```python
from build123d import *
from OCP.BRepFilletAPI import BRepFilletAPI_MakeChamfer

# Parameters (mm, degrees)
BOSS_EXTRUDE1_DEPTH = 37
CUT_EXTRUDE1_REACH  = 150.017
SKETCH2_W           = 42
SKETCH2_H           = 21
SKETCH3_R           = 2
CUT_EXTRUDE2_DEPTH  = 10
FILLET1_R           = 20
CUT_EXTRUDE5_REACH  = 150.017
SKETCH6_W           = 42
SKETCH6_H           = 9
SKETCH7_R           = 2
CUT_EXTRUDE6_DEPTH  = 10
CUT_EXTRUDE7_DEPTH  = 9
SKETCH9_R           = 2
CUT_EXTRUDE8_DEPTH  = 10
CUT_EXTRUDE9_DEPTH  = 6
SKETCH11_R          = 2
CUT_EXTRUDE10_DEPTH = 9
SKETCH12_R          = 2
CUT_EXTRUDE11_DEPTH = 10
CUT_EXTRUDE12_REACH = 140.091
CUT_EXTRUDE16_REACH = 142.222
SKETCH14_W          = 7
SKETCH14_H          = 27
CUT_EXTRUDE17_REACH = 108.34
SKETCH16_W          = 7
SKETCH16_H          = 10
CUT_EXTRUDE18_REACH = 146.306
SKETCH15_W          = 5
SKETCH15_H          = 10
CHAMFER1_SIZE       = 4.5
CHAMFER1_SIZE2      = 7.794228634
CUT_EXTRUDE19_DEPTH = 8


with BuildPart() as part:
    # Sketch1 → Boss-Extrude1 (new body)
    with BuildSketch(Plane(origin=(0, 0, 0), x_dir=(1, 0, 0), z_dir=(0, 1, 0))):
        Polygon((-15.317617866, 43.23325062), (45.682382134, 43.23325062), (45.682382134, -16.76674938), (65.682382134, -16.76674938), (65.682382134, 118.23325062), (45.682382134, 118.23325062), (45.682382134, 58.23325062), (-15.317617866, 58.23325062), align=None)
    extrude(amount=BOSS_EXTRUDE1_DEPTH)

    # Sketch2 → Cut-Extrude1 (cut, up to next)
    with BuildSketch(Plane(origin=(65.682382134, 0, 0), x_dir=(0, 0, -1), z_dir=(1, 0, 0)), mode=Mode.PRIVATE) as cut_extrude1_sk1:
        with Locations((13.23325062, 19.5)):
            Rectangle(SKETCH2_W, SKETCH2_H)
    cut_extrude1_tool1 = extrude(cut_extrude1_sk1.sketch, amount=-CUT_EXTRUDE1_REACH, mode=Mode.PRIVATE) & part.part
    # Sketch2 → Cut-Extrude1 (cut, up to next)
    with BuildSketch(Plane(origin=(65.682382134, 0, 0), x_dir=(0, 0, -1), z_dir=(1, 0, 0)), mode=Mode.PRIVATE) as cut_extrude1_sk2:
        with Locations((88.23325062, 19.5)):
            Rectangle(SKETCH2_W, SKETCH2_H)
    cut_extrude1_tool2 = extrude(cut_extrude1_sk2.sketch, amount=-CUT_EXTRUDE1_REACH, mode=Mode.PRIVATE) & part.part
    add(cut_extrude1_tool1.solids().sort_by_distance((65.682382, 19.5, -13.233251))[0], mode=Mode.SUBTRACT)
    add(cut_extrude1_tool2.solids().sort_by_distance((65.682382, 19.5, -88.233251))[0], mode=Mode.SUBTRACT)

    # Sketch3 → Cut-Extrude2 (cut)
    with BuildSketch(Plane.ZY.offset(-45.682382134)):
        with Locations((11.26674938, 24.75)):
            Circle(SKETCH3_R)
        with Locations((11.26674938, 15.25)):
            Circle(SKETCH3_R)
        with Locations((-37.73325062, 24.75)):
            Circle(SKETCH3_R)
        with Locations((-37.73325062, 15.25)):
            Circle(SKETCH3_R)
        with Locations(Location((-112.73325062, 24.75, 0), (0, 0, 180))):
            Circle(SKETCH3_R)
        with Locations(Location((-112.73325062, 15.25, 0), (0, 0, 180))):
            Circle(SKETCH3_R)
        with Locations(Location((-63.73325062, 15.25, 0), (0, 0, 180))):
            Circle(SKETCH3_R)
        with Locations(Location((-63.73325062, 24.75, 0), (0, 0, 180))):
            Circle(SKETCH3_R)
    extrude(amount=-CUT_EXTRUDE2_DEPTH, mode=Mode.SUBTRACT)

    # Fillet1
    fillet1_edges = [part.edges().sort_by_distance(p)[0] for p in [
        (55.682382134, 0, -118.23325062),
        (55.682382134, 0, 16.76674938),
    ]]
    fillet(fillet1_edges, radius=FILLET1_R)

    # Sketch6 → Cut-Extrude5 (cut, up to next)
    with BuildSketch(Plane(origin=(65.682382134, 0, 0), x_dir=(0, 0, -1), z_dir=(1, 0, 0)), mode=Mode.PRIVATE) as cut_extrude5_sk1:
        with Locations((13.23325062, 4.5)):
            Rectangle(SKETCH6_W, SKETCH6_H)
    cut_extrude5_tool1 = extrude(cut_extrude5_sk1.sketch, amount=-CUT_EXTRUDE5_REACH, mode=Mode.PRIVATE) & part.part
    # Sketch6 → Cut-Extrude5 (cut, up to next)
    with BuildSketch(Plane(origin=(65.682382134, 0, 0), x_dir=(0, 0, -1), z_dir=(1, 0, 0)), mode=Mode.PRIVATE) as cut_extrude5_sk2:
        with Locations((88.23325062, 4.5)):
            Rectangle(SKETCH6_W, SKETCH6_H)
    cut_extrude5_tool2 = extrude(cut_extrude5_sk2.sketch, amount=-CUT_EXTRUDE5_REACH, mode=Mode.PRIVATE) & part.part
    add(cut_extrude5_tool1.solids().sort_by_distance((65.682382, 4.5, -13.233251))[0], mode=Mode.SUBTRACT)
    add(cut_extrude5_tool2.solids().sort_by_distance((65.682382, 4.5, -88.233251))[0], mode=Mode.SUBTRACT)

    # Sketch7 → Cut-Extrude6 (cut)
    with BuildSketch(Plane.ZY.offset(15.317617866)):
        with Locations((-50.73325062, 27)):
            Circle(SKETCH7_R)
        with Locations((-50.73325062, 12)):
            Circle(SKETCH7_R)
    extrude(amount=-CUT_EXTRUDE6_DEPTH, mode=Mode.SUBTRACT)

    # Sketch8 → Cut-Extrude7 (cut)
    with BuildSketch(Plane.XZ):
        Polygon((45.682382134, -67.23325062), (45.682382134, -58.23325062), (25.682382134, -58.23325062), (25.682382134, -43.23325062), (45.682382134, -43.23325062), (45.682382134, -34.23325062), (65.682382134, -34.23325062), (65.682382134, -67.23325062), align=None)
    extrude(amount=-CUT_EXTRUDE7_DEPTH, mode=Mode.SUBTRACT)

    # Sketch9 → Cut-Extrude8 (cut)
    with BuildSketch(Plane.XZ.offset(-9)):
        with Locations(Location((55.682382134, -42.23325062, 0), (0, 0, 270))):
            Circle(SKETCH9_R)
        with Locations(Location((55.682382134, -59.23325062, 0), (0, 0, 270))):
            Circle(SKETCH9_R)
        with Locations(Location((35.682382134, -50.73325062, 0), (0, 0, 270))):
            Circle(SKETCH9_R)
    extrude(amount=-CUT_EXTRUDE8_DEPTH, mode=Mode.SUBTRACT)

    # Sketch10 → Cut-Extrude9 (cut)
    with BuildSketch(Plane(origin=(0, 37, 0), x_dir=(1, 0, 0), z_dir=(0, 1, 0))):
        Polygon((45.682382134, 62.23325062), (65.682382134, 62.23325062), (65.682382134, 39.23325062), (45.682382134, 39.23325062), (45.682382134, 43.23325062), (31.682382134, 43.23325062), (31.682382134, 58.23325062), (45.682382134, 58.23325062), align=None)
    extrude(amount=-CUT_EXTRUDE9_DEPTH, mode=Mode.SUBTRACT)

    # Sketch11 → Cut-Extrude10 (cut)
    with BuildSketch(Plane(origin=(0, 31, 0), x_dir=(1, 0, 0), z_dir=(0, 1, 0))):
        with Locations(Location((39.682382134, 50.73325062, 0), (0, 0, 270))):
            Circle(SKETCH11_R)
    extrude(amount=-CUT_EXTRUDE10_DEPTH, mode=Mode.SUBTRACT)

    # Sketch12 → Cut-Extrude11 (cut)
    with BuildSketch(Plane(origin=(0, 37, 0), x_dir=(1, 0, 0), z_dir=(0, 1, 0))):
        with Locations(Location((60.682382134, -2.76674938, 0), (0, 0, 270))):
            Circle(SKETCH12_R)
        with Locations(Location((60.682382134, 104.23325062, 0), (0, 0, 270))):
            Circle(SKETCH12_R)
    extrude(amount=-CUT_EXTRUDE11_DEPTH, mode=Mode.SUBTRACT)

    # Sketch13 → Cut-Extrude12 (cut, up to next)
    with BuildSketch(Plane.ZY.offset(-45.682382134), mode=Mode.PRIVATE) as cut_extrude12_sk1:
        with BuildLine():
            Line((-111.23325062, 37), (-118.23325062, 37))
            Line((-118.23325062, 37), (-118.23325062, 21.801315846))
            ThreePointArc((-118.23325062, 21.801315846), (-116.399152745, 30.167916112), (-111.23325062, 37))
        make_face()
    cut_extrude12_tool1 = extrude(cut_extrude12_sk1.sketch, amount=-CUT_EXTRUDE12_REACH, mode=Mode.PRIVATE) & part.part
    # Sketch13 → Cut-Extrude12 (cut, up to next)
    with BuildSketch(Plane.ZY.offset(-45.682382134), mode=Mode.PRIVATE) as cut_extrude12_sk2:
        with BuildLine():
            Line((9.76674938, 37), (16.76674938, 37))
            Line((16.76674938, 37), (16.76674938, 21.801315846))
            ThreePointArc((16.76674938, 21.801315846), (14.932651504, 30.167916112), (9.76674938, 37))
        make_face()
    cut_extrude12_tool2 = extrude(cut_extrude12_sk2.sketch, amount=-CUT_EXTRUDE12_REACH, mode=Mode.PRIVATE) & part.part
    add(cut_extrude12_tool1.solids().sort_by_distance((45.682382, 33.346132, -116.215792))[0], mode=Mode.SUBTRACT)
    add(cut_extrude12_tool2.solids().sort_by_distance((45.682382, 33.346132, 14.749291))[0], mode=Mode.SUBTRACT)

    # Sketch14 → Cut-Extrude16 (cut, up to next)
    with BuildSketch(Plane(origin=(0, 37, 0), x_dir=(1, 0, 0), z_dir=(0, 1, 0)), mode=Mode.PRIVATE) as cut_extrude16_sk1:
        with Locations((62.182382134, 50.73325062)):
            Rectangle(SKETCH14_W, SKETCH14_H)
    cut_extrude16_tool1 = extrude(cut_extrude16_sk1.sketch, amount=-CUT_EXTRUDE16_REACH, mode=Mode.PRIVATE) & part.part
    add(cut_extrude16_tool1.solids().sort_by_distance((62.182382, 37, -50.733251))[0], mode=Mode.SUBTRACT)

    # Sketch16 → Cut-Extrude17 (cut, up to next)
    with BuildSketch(Plane.XY.offset(-43.23325062), mode=Mode.PRIVATE) as cut_extrude17_sk1:
        with Locations((28.182382134, 20)):
            Rectangle(SKETCH16_W, SKETCH16_H)
    cut_extrude17_tool1 = extrude(cut_extrude17_sk1.sketch, amount=-CUT_EXTRUDE17_REACH, mode=Mode.PRIVATE) & part.part
    add(cut_extrude17_tool1.solids().sort_by_distance((28.182382, 20, -43.233251))[0], mode=Mode.SUBTRACT)

    # Sketch15 → Cut-Extrude18 (cut, up to next)
    with BuildSketch(Plane(origin=(58.682382134, 0, 0), x_dir=(0, 0, -1), z_dir=(1, 0, 0)), mode=Mode.PRIVATE) as cut_extrude18_sk1:
        with Locations((50.73325062, 20)):
            Rectangle(SKETCH15_W, SKETCH15_H)
    cut_extrude18_tool1 = extrude(cut_extrude18_sk1.sketch, amount=-CUT_EXTRUDE18_REACH, mode=Mode.PRIVATE) & part.part
    add(cut_extrude18_tool1.solids().sort_by_distance((58.682382, 20, -50.733251))[0], mode=Mode.SUBTRACT)

    # Chamfer1: one chamfer whose edges measure the first distance from different faces: ONE call of the kernel's chamfer builder (chamfer() names one face for all edges)
    chamfer1_edges_1 = [part.edges().sort_by_distance(p)[0] for p in [
        (31.682382134, 20, -53.23325062),
    ]]
    chamfer1_side_1 = [part.faces().sort_by_distance(p)[0] for p in [
        (31.682382134, 20, -55.73325062),
    ]]
    chamfer1_edges_2 = [part.edges().sort_by_distance(p)[0] for p in [
        (31.682382134, 20, -48.23325062),
    ]]
    chamfer1_side_2 = [part.faces().sort_by_distance(p)[0] for p in [
        (31.682382134, 20, -45.73325062),
    ]]
    chamfer1 = BRepFilletAPI_MakeChamfer(part.part.solid().wrapped)
    for e in chamfer1_edges_1:
        chamfer1.Add(CHAMFER1_SIZE, CHAMFER1_SIZE2, e.wrapped, chamfer1_side_1[0].wrapped)  # the first distance lies on this face
    for e in chamfer1_edges_2:
        chamfer1.Add(CHAMFER1_SIZE, CHAMFER1_SIZE2, e.wrapped, chamfer1_side_2[0].wrapped)  # the first distance lies on this face
    add(Compound.cast(chamfer1.Shape()), mode=Mode.REPLACE)

    # Sketch18 → Cut-Extrude19 (cut)
    with BuildSketch(Plane(origin=(65.682382134, 0, 0), x_dir=(0, 0, -1), z_dir=(1, 0, 0))):
        with BuildLine():
            Line((109.23325062, 25.296706912), (112.23325062, 25.296706912))
            Line((112.23325062, 25.296706912), (114.23325062, 22.989626664))
            Line((114.23325062, 22.989626664), (114.23325062, 10.989626664))
            ThreePointArc((114.23325062, 10.989626664), (112.030073944, 7.882471629), (109.23325062, 5.296706912))
            Line((109.23325062, 5.296706912), (109.23325062, 25.296706912))
        make_face()
        with BuildLine():
            Line((-7.763672274, 25.296706912), (-7.763672274, 5.296706912))
            ThreePointArc((-7.763672274, 5.296706912), (-10.560495598, 7.882471629), (-12.763672274, 10.989626664))
            Line((-12.763672274, 10.989626664), (-12.763672274, 22.989626664))
            Line((-12.763672274, 22.989626664), (-10.763672274, 25.296706912))
            Line((-10.763672274, 25.296706912), (-7.763672274, 25.296706912))
        make_face()
    extrude(amount=-CUT_EXTRUDE19_DEPTH, mode=Mode.SUBTRACT)


solid = part.part
```
The listing builds one solid part. Answer for the finished solid, in the listing's coordinates (mm). A direction names the side the tool comes from. Give positions to 0.01 mm unless a question says otherwise; leave off trailing zeros. Order: outer loops, then holes, each group sorted by start corner. A loop starts at its lowest first (then second) coordinate and runs counter-clockwise, first axis right, second up.
1) Given P1, Ø6.5, axis at x = 55.68, z = -42.23, coming from the -Y side; P2, Ø0.9, axis at x = 62.5, z = -110, coming from the -Y side; P3, Ø5, axis at x = 35.68, z = -50.73, coming from the +Y side, each flat-ended and moving along its own axis, determine where each tip first touches the part or whether it passes through.
Reported:
P1: stops at y = 9
P2: stops at y = 3.51
P3: stops at y = 31
2) Consider line 1 along Z through (x, y) = (56, 21); line 2 along Z through (x, y) = (53.5, 12.5); line 3 along Y through (x, z) = (47.5, -36.5). Determine where each line is inside the solid, lowest interval first.
Reported:
line 1: z = -118.23 to -109.23, -67.23 to -53.23, -48.23 to -34.23, 7.77 to 16.77
line 2: z = -116.77 to -109.23, -67.23 to -34.23, 7.77 to 15.31
line 3: y = 9 to 13.68, 16.82 to 23.18, 26.32 to 37
3) Find section D-D on z = -72. Write down the section's boundary in (x, y).
Reported:
outline: (45.68, 30) - (65.68, 30) - (65.68, 37) - (45.68, 37) - close
4) Find section A-A on x = 51. Give the number of separate pieces and of enclosed holes in the cut face, then the cut area to 3 significant figures.
Reported:
separate pieces: 1
enclosed holes: 9
area: 1,680 mm2
5) Determine the mould class of faces 4 (the face through (5, 0, -51)), 5 (the face through (38.465, 28.042, -52.32)), 6 (the face through (62, 17, -114.233)) for opening direction Y: pulls with the +Y half, pulls with the -Y half, needs draft (parallel to the pull), parting line crosses it, or undercut.
Reported:
face 4: pulls with the -Y half
face 5: needs draft
face 6: undercut
6) Find section B-B on y = 32.5. Write down the section's boundary in (x, z).
Reported:
outline: (-15.32, -58.23) - (31.68, -58.23) - (31.68, -43.23) - (-15.32, -43.23) - close; (45.68, -115.13) - (65.68, -115.13) - (65.68, -64.23) - (58.68, -64.23) - (58.68, -62.23) - (45.68, -62.23) - close; (45.68, -39.23) - (58.68, -39.23) - (58.68, -37.23) - (65.68, -37.23) - (65.68, 13.66) - (45.68, 13.66) - close; hole circle Ø4 at (60.68, -104.23); hole circle Ø4 at (60.68, 2.77)
7) Find section C-C on y = 7. Write down the section's boundary in (x, z), then the cut area to 3 significant figures.
Reported:
outline: (-15.32, -58.23) - (25.68, -58.23) - (25.68, -43.23) - (-15.32, -43.23) - close; (45.68, -113.43) - (65.68, -113.43) - (65.68, -111.2) - (57.68, -111.2) - (57.68, -109.23) - (45.68, -109.23) - close; (45.68, 7.77) - (57.68, 7.77) - (57.68, 9.73) - (65.68, 9.73) - (65.68, 11.97) - (45.68, 11.97) - close
area: 751 mm2
8) For faces 1 (the face through (25.682, 4, -51)), 2 (the face through (15, 18, -43.233)), 3 (the face through (62, 17, 12.764)), determine the directions among +Z, -Z, +X, -X, +Y, -Y from which every point of the face is accessible in a straight line to the end or side of a thin tool.
Reported:
face 1: +Z, -Z, +X, -Y
face 2: +Z, -X, +Y, -Y
face 3: +X
